from build123d import *

# Parameters (mm, degrees)
F0_R      = 1.778
F1_DEPTH  = 17.78
F3_R      = 1.778
F4_DEPTH  = 16.002
F2_R      = 1.27
F5_DEPTH  = 25.4
F7_DEPTH  = 2.54
F8_W      = 16.9942029752
F8_H      = 1.524
F8_H_2    = 3.048
F9_DEPTH  = 5.08
F11_DEPTH = 13.462
F12_R     = 2.54


# Not quite as in the source:
# - a feature names something its author has since deleted; it is built from what else it names


with BuildPart() as f1:
    # F0 (on Front) → F1 (new body)
    with BuildSketch(Plane.XZ):
        with BuildLine():
            Line((-21.7745867558, 0), (-5.7350052521, 0))
            Line((-5.7350052521, 0), (-4.7625, 0))
            ThreePointArc((-4.7625, 0), (-3.3675960454, 3.3675960454), (0, 4.7625))
            Line((0, 4.7625), (0, 7.4168))
            Line((0, 7.4168), (-21.7745867558, 7.4168))
            Line((-21.7745867558, 7.4168), (-21.7745867558, 5.8928))
            Line((-21.7745867558, 5.8928), (-3.9945867558, 5.8928))
            Line((-3.9945867558, 5.8928), (-3.9945867558, 3.048))
            Line((-3.9945867558, 3.048), (-21.7745867558, 3.048))
            Line((-21.7745867558, 3.048), (-21.7745867558, 0))
        make_face()
        with BuildLine():
            ThreePointArc((4.7625, 0), (4.4508557537, -1.6944879196), (3.5567092138, -3.1672110474))
            Line((3.5567092138, -3.1672110474), (51.8252535905, -11.7928625561))
            ThreePointArc((51.8252535905, -11.7928625561), (51.6705317006, -8.7770103), (53.3605608921, -6.2743906673))
            Line((53.3605608921, -6.2743906673), (4.0277059432, 2.5414545216))
            ThreePointArc((4.0277059432, 2.5414545216), (4.5751150698, 1.3227729767), (4.7625, 0))
        make_face()
        with BuildLine():
            ThreePointArc((0, 4.7625), (-3.3675960454, 3.3675960454), (-4.7625, 0))
            ThreePointArc((-4.7625, 0), (-1.6944879196, -4.4508557537), (3.5567092138, -3.1672110474))
            ThreePointArc((3.5567092138, -3.1672110474), (4.4508557537, -1.6944879196), (4.7625, 0))
            ThreePointArc((4.7625, 0), (4.5751150698, 1.3227729767), (4.0277059432, 2.5414545216))
            ThreePointArc((4.0277059432, 2.5414545216), (2.2997531488, 4.1704366324), (0, 4.7625))
        make_face()
        Circle(F0_R, mode=Mode.SUBTRACT)
        with BuildLine():
            ThreePointArc((53.3605608921, -6.2743906673), (51.6705317006, -8.7770103), (51.8252535905, -11.7928625561))
            ThreePointArc((51.8252535905, -11.7928625561), (57.1438640566, -14.7330470759), (61.0212711223, -10.0535153956))
            ThreePointArc((61.0212711223, -10.0535153956), (58.3657452594, -5.7824422007), (53.3605608921, -6.2743906673))
        make_face()
        with Locations((56.2587711223, -10.0535153956)):
            Circle(F0_R, mode=Mode.SUBTRACT)
    extrude(amount=F1_DEPTH)

    # F3 (on face) → F4 (cut)
    with BuildSketch(Plane.XZ.offset(17.78)):
        with BuildLine():
            ThreePointArc((4.0277059432, 2.5414545216), (2.2997531488, 4.1704366324), (0, 4.7625))
            ThreePointArc((0, 4.7625), (-3.3675960454, 3.3675960454), (-4.7625, 0))
            ThreePointArc((-4.7625, 0), (-4.5665768899, -1.3519547915), (-3.994927608, -2.5926742288))
            ThreePointArc((-3.994927608, -2.5926742288), (-0.3612920968, -4.7487760813), (3.5567092138, -3.1672110474))
            Line((3.5567092138, -3.1672110474), (51.8252535905, -11.7928625561))
            ThreePointArc((51.8252535905, -11.7928625561), (60.847010544, -11.3300204911), (53.3605608921, -6.2743906673))
            Line((53.3605608921, -6.2743906673), (4.0277059432, 2.5414545216))
        make_face()
        with Locations((56.2587711223, -10.0535153956)):
            Circle(F3_R, mode=Mode.SUBTRACT)
        Circle(F3_R, mode=Mode.SUBTRACT)
    extrude(amount=-F4_DEPTH, mode=Mode.SUBTRACT)

    # F2 (on face) → F5 (cut)
    with BuildSketch(Plane.XY.offset(7.4168)):
        with Locations((-9.1804936528, -10.1120751351)):
            Circle(F2_R)
    extrude(amount=-F5_DEPTH, mode=Mode.SUBTRACT)

    # F6 (on face) → F7 (cut)
    with BuildSketch(Plane.XZ.offset(17.78)):
        with BuildLine():
            Line((-21.7745867558, 0), (-4.7625, 0))
            ThreePointArc((-4.7625, 0), (-3.3675960454, 3.3675960454), (0, 4.7625))
            Line((0, 4.7625), (0, 7.4168))
            Line((0, 7.4168), (-21.7745867558, 7.4168))
            Line((-21.7745867558, 7.4168), (-21.7745867558, 5.8928))
            Line((-21.7745867558, 5.8928), (-3.9945867558, 5.8928))
            Line((-3.9945867558, 5.8928), (-3.9945867558, 3.048))
            Line((-3.9945867558, 3.048), (-21.7745867558, 3.048))
            Line((-21.7745867558, 3.048), (-21.7745867558, 0))
        make_face()
    extrude(amount=-F7_DEPTH, mode=Mode.SUBTRACT)

    # F8 (on face) → F9 (cut)
    with BuildSketch(Plane(origin=(0, 0, 0), x_dir=(-1, 0, 0), z_dir=(0, 1, 0))):
        with Locations((13.2774852682, 6.6548)):
            Rectangle(F8_W, F8_H)
        with Locations((13.2774852682, 1.524)):
            Rectangle(F8_W, F8_H_2)
    extrude(amount=-F9_DEPTH, mode=Mode.SUBTRACT)

    # F10 (on face) → F11 (join, through all)
    with BuildSketch(Plane.XZ.offset(1.778)):
        with BuildLine():
            ThreePointArc((-3.8153238056, 0), (-2.6978413354, 2.6978413354), (0, 3.8153238056))
            Line((0, 3.8153238056), (0, 4.7625))
            ThreePointArc((0, 4.7625), (-3.3675960454, 3.3675960454), (-4.7625, 0))
            Line((-4.7625, 0), (-3.8153238056, 0))
        make_face()
        with BuildLine():
            Line((-4.2348116803, -2.1789392561), (-3.434889127, -1.6607927104))
            ThreePointArc((-3.434889127, -1.6607927104), (-3.7189991932, -0.8519041865), (-3.8153238056, 0))
            Line((-3.8153238056, 0), (-4.7625, 0))
            ThreePointArc((-4.7625, 0), (-4.6286983525, -1.1209628946), (-4.2348116803, -2.1789392561))
        make_face()
    extrude(amount=F11_DEPTH)

    # F12
    f12_edges = [f1.edges().sort_by_distance(p)[0] for p in [
        (-4.780384, -5.08, 1.524),
        (-4.780384, -5.08, 6.6548),
    ]]
    fillet(f12_edges, radius=F12_R)


solid = f1.part
Geometry: final body of the model. Coordinates: model frame, mm. A direction names the side the tool comes from. Round coordinates to 2 decimals unless told otherwise and drop trailing zeros. Loops run counter-clockwise (first coordinate to the right, second up) from the corner with the lowest first, then second, coordinate; pieces in that order, holes last.
Q1. Material intervals for L1, parallel to Z at x = -5.5, y = -6; L2, parallel to Y at x = 2, z = -3; L3, parallel to X at y = -13.75, z = 4.25, sorted ascending.
Q2. Section D-D on x = 55.5. Return loops of the section in (y, z), plus the area to 3 significant figures.
Q3. Section B-B on x = -1. Return loops of the section in (y, z).
Q4. Access query for faces 5 (the flat face through (26, 0, -4)), 6 (the flat face through (-13, -9, 3.048)), 7 (the flat face through (-14, -5.08, 2)). Directions: +Z, -Z, +X, -X, +Y, -Y. A direction counts if a zero-diameter tool reaches every point of the face in a straight line with its end or side. Return the directions, or none.
Q5. Pin query (flat end, axial travel): P1, Ø7.5, axis at x = -17, y = -9, coming from the -Z side; P2, Ø3.5, axis at x = -12, z = 1, coming from the +Y side; P3, Ø3, axis at x = 0, z = 0, coming from the -Y side; P4, Ø1.2, axis at y = -1, z = 7, coming from the -X side. Return the tip coordinate at first contact, or that it passes through.
Q6. Pull-direction query (Z, two-part tool) for faces 1 (the flat face through (-11, -15.24, 2.7)), 2 (the flat face through (29.04, -0.88, -1.93)), 3 (the flat face through (27.35, -0.88, -7.42)), 4 (the flat face through (-13, -9, 5.893)); classes: released by +Z, released by -Z, zero draft, split by the parting line, or undercut.
Q7. Section C-C on y = -6.75. Return loops of the section in (x, z) (1 decimal).
Q8. Section A-A on y = -1. State how many separate pieces and enclosed holes the cut face has, plus the area to 3 significant figures.
Evaluation:
1. L1: z = 0 to 3.05, 5.89 to 7.42
1. L2: y = -1.78 to 0
1. L3: x = -3.99 to 0
2. outline: (-1.78, -14.76) - (0, -14.76) - (0, -11.66) - (-1.78, -11.66) - close; (-1.78, -8.45) - (0, -8.45) - (0, -5.35) - (-1.78, -5.35) - close
2. area: 11.0 mm2
3. outline: (-15.24, 3.68) - (-1.78, 3.68) - (-1.78, 1.47) - (0, 1.47) - (0, 7.42) - (-15.24, 7.42) - close; (-1.78, -4.66) - (0, -4.66) - (0, -1.47) - (-1.78, -1.47) - close
4. face 5: +Z, -Z, +X, -X, +Y
4. face 6: -X, +Y, -Y
4. face 7: +Z, -Z, -X, +Y
5. P1: stops at z = 0
5. P2: stops at y = -5.08
5. P3: passes through
5. P4: stops at x = -4.78
6. face 1: zero draft
6. face 2: released by +Z
6. face 3: released by -Z
6. face 4: undercut
7. outline: (-21.8, 0) - (-4.8, 0) arc R4.8 ccw to (-4.2, -2.2) - (-3.4, -1.7) arc R3.8 cw to (0, 3.8) - (0, 7.4) - (-21.8, 7.4) - (-21.8, 5.9) - (-4, 5.9) - (-4, 3) - (-21.8, 3) - close
8. separate pieces: 1
8. enclosed holes: 2
8. area: 413 mm2
